Design review of the part built by this model. Coordinates are the model's own, in mm. A direction names the side the tool comes from. Give positions to 0.01 mm unless a question says otherwise; leave off trailing zeros. Loops run counter-clockwise (first coordinate to the right, second up) from the corner with the lowest first, then second, coordinate; pieces in that order, holes last. Notation, with made-up numbers: (83, -23.5) - (93, -23.5) arc R26 ccw to (93, 10.5) - close; hole circle Ø8 at (14, 73.5). An arc over 180 degrees is marked (long way). Write each question's results on one line, items separated by ' | '.
```python
from build123d import *

# Parameters (mm, degrees)
SKETCH1_W           = 1905
SKETCH1_H           = 1270
BOSS_EXTRUDE1_DEPTH = 5.08
BOSS_EXTRUDE2_DEPTH = 228.6


with BuildPart() as part:
    # Sketch1 → Boss-Extrude1 (new body)
    with BuildSketch(Plane(origin=(0, 0, 0), x_dir=(1, 0, 0), z_dir=(0, 1, 0))):
        Rectangle(SKETCH1_W, SKETCH1_H)
    extrude(amount=BOSS_EXTRUDE1_DEPTH)

    # Sketch2 → Boss-Extrude2 (add, symmetric)
    with BuildSketch(Plane.XY):
        Polygon((194.31, 5.08), (194.31, 49.53), (270.129, 49.53), (270.129, 93.98), (345.948, 93.98), (345.948, 138.43), (421.767, 138.43), (421.767, 182.88), (497.586, 182.88), (497.586, 227.33), (573.405, 227.33), (573.405, 271.78), (649.224, 271.78), (649.224, 316.23), (725.043, 316.23), (725.043, 360.68), (800.862, 360.68), (800.862, 405.13), (876.681, 405.13), (876.681, 449.58), (952.5, 449.58), (952.5, 5.08), align=None)
    extrude(amount=BOSS_EXTRUDE2_DEPTH, both=True)


solid = part.part
```
Item 1: We need section D-D on z = 321. Give the boundary of the cut face in (x, y), then the cut area to 3 significant figures.
Output values:
outline: (-952.5, 0) - (952.5, 0) - (952.5, 5.08) - (-952.5, 5.08) - close | area: 9,680 mm²
Item 2: Wall thickness on probe 1 along Y at (x, z) = (661, 192); probe 2 along Z at (x, y) = (615.5, 262); probe 3 along Y at (x, z) = (-653.5, 569): over which ranges is each line inside the solid? List them lowest first.
Output values:
probe 1: y = 0 to 316.23 | probe 2: z = -228.6 to 228.6 | probe 3: y = 0 to 5.08
Item 3: Tool access review of faces 1 (the face through (663, 181, 228.6)), 2 (the face through (383, 138.43, 3)), 3 (the face through (-13, 0, -9)): name each direction out of +Z, -Z, +X, -X, +Y, -Y from which nothing blocks a thin tool from reaching the whole face with its end or side.
Output values:
face 1: +Z, +X, -X, +Y | face 2: +Z, -Z, -X, +Y | face 3: +Z, -Z, +X, -X, -Y
Item 4: We need section B-B on z = -183.5. Give the boundary of the cut face in (x, y) (3 decimals).
Output values:
outline: (-952.5, 0) - (952.5, 0) - (952.5, 449.58) - (876.681, 449.58) - (876.681, 405.13) - (800.862, 405.13) - (800.862, 360.68) - (725.043, 360.68) - (725.043, 316.23) - (649.224, 316.23) - (649.224, 271.78) - (573.405, 271.78) - (573.405, 227.33) - (497.586, 227.33) - (497.586, 182.88) - (421.767, 182.88) - (421.767, 138.43) - (345.948, 138.43) - (345.948, 93.98) - (270.129, 93.98) - (270.129, 49.53) - (194.31, 49.53) - (194.31, 5.08) - (-952.5, 5.08) - close
Item 5: Clearance check with flat-ended pins moving along their axes: P1, Ø1.5, axis at x = 743.5, y = 203.5, coming from the -Z side; P2, Ø1, axis at x = -15.5, z = -391, coming from the +Y side; P3, Ø22.5, axis at x = 705.5, z = 16, coming from the +Y side. State where each tip first meets the part, or that it passes through.
Output values:
P1: stops at z = -228.6 | P2: stops at y = 5.08 | P3: stops at y = 316.23
Item 6: We need section A-A on x = 701. Give the boundary of the cut face in (y, z).
Output values:
outline: (0, -635) - (5.08, -635) - (5.08, -228.6) - (316.23, -228.6) - (316.23, 228.6) - (5.08, 228.6) - (5.08, 635) - (0, 635) - close
Item 7: We need section C-C on x = 384. Give the boundary of the cut face in (y, z).
Output values:
outline: (0, -635) - (5.08, -635) - (5.08, -228.6) - (138.43, -228.6) - (138.43, 228.6) - (5.08, 228.6) - (5.08, 635) - (0, 635) - close
